Input: part model. Units: mm. Frame: model coordinates. Round coordinates to 2 decimals unless told otherwise and drop trailing zeros. Loops run counter-clockwise (first coordinate to the right, second up) from the corner with the lowest first, then second, coordinate; pieces in that order, holes last. Notation, with made-up numbers: M 31.25,37.25 L 71.25,37.25 A34 ccw 71.25,76.25 Z; hole C 65,59.5 d1. An arc over 180 degrees is marked long. Put each result on its own line as item: value. Start each with the question number.
1) Pin query (flat end, axial travel): pin 1 (1.5 mm diameter, centred on y = 1.5, z = -48.5, fed in from +X); pin 2 (0.9 mm diameter, centred on x = -134, y = 1.5, fed in from -Z); pin 3 (4 mm diameter, centred on x = 10, z = 24, fed in from -Y); pin 4 (1 mm diameter, centred on y = 1.5, z = -101.5, fed in from +X). Return the tip coordinate at first contact, or that it passes through.
2) Section C-C on x = 27.5. Output: boundary loops of the cut face in (y, z), plus the area to 4 significant figures.
3) Section A-A on y = 1.2. State how many separate pieces and enclosed holes the cut face has, plus the area to 3 significant figures.
4) Section B-B on x = -50.5. Output: boundary loops of the cut face in (y, z).
5) Line query: probe 1 along Z at (x, y) = (-120.5, 0.25); probe 2 along Z at (x, y) = (-126, 1.85); probe 3 along X at (y, z) = (2.45, -27). Output: solid intervals per line, ascending.
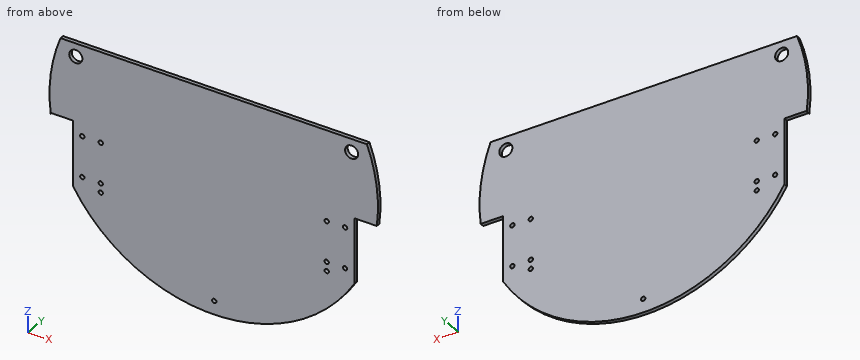
from build123d import *

# Parameters (mm, degrees)
SKETCH2_R           = 125
BOSS_EXTRUDE1_DEPTH = 3
CUT_EXTRUDE1_DEPTH  = 3
SKETCH4_R           = 1.65
SKETCH4_R_2         = 5
CUT_EXTRUDE2_DEPTH  = 10
SKETCH6_R           = 1.65
CUT_EXTRUDE3_DEPTH  = 100


with BuildPart() as part:
    # Sketch2 → Boss-Extrude1 (new body)
    with BuildSketch(Plane(origin=(0, 0, 0), x_dir=(1, 0, 0), z_dir=(0, 1, 0))):
        with Locations((-17.80765369, -0.854894607)):
            Circle(SKETCH2_R)
    extrude(amount=BOSS_EXTRUDE1_DEPTH)

    # Sketch3 → Cut-Extrude1 (cut)
    with BuildSketch(Plane.XZ):
        Polygon((-735.289651923, 45.854894607), (-134.426691587, 45.854894607), (98.811384207, 45.854894607), (699.674344543, 45.854894607), (699.674344543, 1247.580815278), (-735.289651923, 1247.580815278), align=None)
    extrude(amount=-CUT_EXTRUDE1_DEPTH, mode=Mode.SUBTRACT)

    # Sketch4 → Cut-Extrude2 (cut)
    with BuildSketch(Plane(origin=(0, 0, 0), x_dir=(-1, 0, 0), z_dir=(0, -1, 0))):
        with Locations((117.80765369, 54.145105393)):
            Circle(SKETCH4_R)
        with Locations((117.881226527, 23.145192699)):
            Circle(SKETCH4_R)
        with Locations((103.80765369, 54.145105393)):
            Circle(SKETCH4_R)
        with Locations((103.80765369, 23.145105393)):
            Circle(SKETCH4_R)
        with Locations((-68.19234631, 54.267083079)):
            Circle(SKETCH4_R)
        with Locations((-82.19234631, 54.267083079)):
            Circle(SKETCH4_R)
        with Locations((-82.19234631, 23.267083079)):
            Circle(SKETCH4_R)
        with Locations((-68.19234631, 23.267083079)):
            Circle(SKETCH4_R)
        with Locations((122.80765369, -35.854894607)):
            Circle(SKETCH4_R_2)
        with Locations((-87.19234631, -35.854894607)):
            Circle(SKETCH4_R_2)
        Polygon((124.881226527, 63.645105393), (124.881226527, 13.645105393), (141.357501756, 13.645105393), (159.377606719, 40.481299306), align=None)
        Polygon((-89.19234631, 63.767083079), (-89.19234631, 13.767083079), (-106.334191667, 13.767083079), (-114.079843912, 54.596315864), align=None)
    extrude(amount=-CUT_EXTRUDE2_DEPTH, mode=Mode.SUBTRACT)

    # Sketch6 → Cut-Extrude3 (cut)
    with BuildSketch(Plane(origin=(0, 0, 0), x_dir=(-1, 0, 0), z_dir=(0, -1, 0))):
        with Locations((103.80765369, 61.145105393)):
            Circle(SKETCH6_R)
        with Locations((-68.19234631, 61.267083079)):
            Circle(SKETCH6_R)
        with Locations((17.381226527, 113.706374405)):
            Circle(SKETCH6_R)
    extrude(amount=-CUT_EXTRUDE3_DEPTH, mode=Mode.SUBTRACT)


solid = part.part
Geometry results:
1. pin 1: stops at x = 89.19
1. pin 2: stops at z = -13.65
1. pin 3: stops at y = 0
1. pin 4: stops at x = 54.65
2. outline: M 0,-115.64 L 3,-115.64 L 3,45.85 L 0,45.85 Z
2. area: 484.5 mm²
3. separate pieces: 1
3. enclosed holes: 13
3. area: 34,200 mm²
4. outline: M 0,-119.79 L 3,-119.79 L 3,45.85 L 0,45.85 Z
5. probe 1: z = -70.41 to 31.42, 40.29 to 45.85
5. probe 2: z = -13.65 to 32.01, 39.7 to 45.85
5. probe 3: x = -124.88 to 89.19
